Part model, mm, in its own coordinate system. A direction names the side the tool comes from. Coordinates: 2 decimals unless noted, no trailing zeros. Write each loop counter-clockwise with the first axis right and the second up, starting at its lowest first coordinate (ties: lowest second). Pieces come first, ordered by that corner, then holes. Notation, with made-up numbers: (-34.75, 10) - (-26.75, 10) arc R20 ccw to (-26.75, 42) - close; hole circle Ø8 at (54.5, -34). An arc over 180 degrees is marked (long way). Write each question's results on one line, items separated by ' | '.
from build123d import *

# Parameters (mm, degrees)
F0_W     = 60
F0_H     = 60
F1_DEPTH = 400
F2_W     = 20
F2_H     = 20
F3_DEPTH = 40
F4_W     = 20
F4_H     = 40
F5_DEPTH = 40
F6_W     = 20
F6_H     = 40
F7_DEPTH = 40


with BuildPart() as f1:
    # F0 (on Top) → F1 (new body)
    with BuildSketch(Plane.XY):
        with Locations((-32.3275837302, -19.2534299031)):
            Rectangle(F0_W, F0_H)
    extrude(amount=-F1_DEPTH)

    # F2 (on face) → F3 (cut)
    with BuildSketch(Plane.XY):
        with Locations((-32.3275837302, -19.2534299031)):
            Rectangle(F2_W, F2_H)
        with Locations((-52.3275837302, -19.2534299031)):
            Rectangle(F2_W, F2_H)
        with Locations((-32.3275837302, 0.7465700969)):
            Rectangle(F2_W, F2_H)
        with Locations((-12.3275837302, -19.2534299031)):
            Rectangle(F2_W, F2_H)
        with Locations((-32.3275837302, -39.2534299031)):
            Rectangle(F2_W, F2_H)
    extrude(amount=-F3_DEPTH, mode=Mode.SUBTRACT)

    # F4 (on face) → F5 (cut)
    with BuildSketch(Plane.XZ.offset(49.2534299031)):
        with Locations((-32.3275837302, -300)):
            Rectangle(F4_W, F4_H)
    extrude(amount=-F5_DEPTH, mode=Mode.SUBTRACT)

    # F6 (on face) → F7 (cut)
    with BuildSketch(Plane.YZ.offset(-2.3275837302)):
        with Locations((-19.2534299031, -300)):
            Rectangle(F6_W, F6_H)
    extrude(amount=-F7_DEPTH, mode=Mode.SUBTRACT)


solid = f1.part
(1) Two-plate mould, pull along Y, no slides. Class faces 5 (the flat face through (-33, 10.747, -197)), 6 (the flat face through (-2.328, -20, -197)), 7 (the flat face through (-12, -29.253, -300)): released by +Y, released by -Y, zero draft, split by the parting line, or undercut.
Return value:
face 5: released by +Y | face 6: zero draft | face 7: undercut
(2) Wall check: line 1 (Z direction, x = -40, y = -11); line 2 (X direction, y = -35, z = -310); line 3 (Y direction, x = -7, z = -307). Give the ranges that are in metal, low to high. Write a range as from..to.
Return value:
line 1: z = -400..-320, -280..-40 | line 2: x = -62.33..-42.33, -22.33..-2.33 | line 3: y = -49.25..-29.25, -9.25..10.75
(3) 3-axis set-ups, long thin cutter, end or side, ignore diameter. For faces 1 (the flat face through (-22, -9.253, -300)), 2 (the flat face through (-27, -25, -280)), 3 (the flat face through (-12, -9.253, -20)), 4 (the flat face through (-42.328, -39, -20)): which of +Z, -Z, +X, -X, +Y, -Y reach the whole face in a straight line?
Return value:
face 1: +X | face 2: none | face 3: +Z, +X, -X | face 4: +Z, +Y, -Y
(4) Saw through at D-D on x = -33. Write the cut outline in (y, z).
Return value:
outline: (-49.25, -400) - (10.75, -400) - (10.75, -40) - (-49.25, -40) - (-49.25, -280) - (-9.25, -280) - (-9.25, -320) - (-49.25, -320) - close
(5) Saw through at B-B on x = -10. Write the cut outline in (y, z).
Return value:
outline: (-49.25, -400) - (10.75, -400) - (10.75, 0) - (-9.25, 0) - (-9.25, -40) - (-29.25, -40) - (-29.25, 0) - (-49.25, 0) - close; hole (-29.25, -320) - (-9.25, -320) - (-9.25, -280) - (-29.25, -280) - close
(6) Flat gauge pin, fed straight in: P1, Ø2, axis at x = -34.5, y = -7, coming from the +Z side. Where does the tip first touch, or does it go through?
Return value:
P1: stops at z = -40
(7) Saw through at C-C on y = -18. Write the cut outline in (x, z).
Return value:
outline: (-62.33, -400) - (-2.33, -400) - (-2.33, -320) - (-42.33, -320) - (-42.33, -280) - (-2.33, -280) - (-2.33, -40) - (-62.33, -40) - close
(8) Saw through at A-A on y = -44. Write the cut outline in (x, z).
Return value:
outline: (-62.33, -400) - (-2.33, -400) - (-2.33, 0) - (-22.33, 0) - (-22.33, -40) - (-42.33, -40) - (-42.33, 0) - (-62.33, 0) - close; hole (-42.33, -320) - (-22.33, -320) - (-22.33, -280) - (-42.33, -280) - close
